Design review of the part built by this model. Coordinates are the model's own, in mm. A direction names the side the tool comes from. Coordinates: 2 decimals unless noted, no trailing zeros. Loops run counter-clockwise (first coordinate to the right, second up) from the corner with the lowest first, then second, coordinate; pieces in that order, holes last.
from build123d import *

# Parameters (mm, degrees)
BOSS_EXTRUDE1_DEPTH      = 7.62
BOSS_EXTRUDE2_DEPTH      = 31.75
BOSS_EXTRUDE2_DEPTH_BACK = 38.1
SKETCH2_W                = 25.4
SKETCH2_H                = 6.985
BOSS_EXTRUDE3_START      = -7.62
BOSS_EXTRUDE3_DEPTH      = 7.62
SKETCH4_R                = 3.175
CUT_EXTRUDE1_DEPTH       = 7.62
CHAMFER1_SIZE            = 8.89
FILLET1_R                = 6.35
FILLET2_R                = 5.08


with BuildPart() as part:
    # Sketch1 → Boss-Extrude1 (new body)
    with BuildSketch(Plane.XY):
        with BuildLine():
            Line((41.275, -41.275), (0, -41.275))
            ThreePointArc((0, -41.275), (-40.972302797, -4.989592018), (-9.906, 40.068650951))
            Line((-9.906, 40.068650951), (-9.906, 0))
            ThreePointArc((-9.906, 0), (0, -9.906), (9.906, 0))
            Line((9.906, 0), (9.906, 40.068650951))
            ThreePointArc((9.906, 40.068650951), (32.4999675, 25.443618797), (41.275, 0))
            Line((41.275, 0), (41.275, -41.275))
        make_face()
    extrude(amount=BOSS_EXTRUDE1_DEPTH)

    # Sketch2 → Boss-Extrude2 (add, two sides: drawn at the far end of the back side and taken through both)
    with BuildSketch(Plane.XY.offset(7.62).offset(-BOSS_EXTRUDE2_DEPTH_BACK)):
        with Locations((28.575, -41.5925)):
            Rectangle(SKETCH2_W, SKETCH2_H)
    extrude(amount=BOSS_EXTRUDE2_DEPTH + BOSS_EXTRUDE2_DEPTH_BACK)

    # Sketch3 → Boss-Extrude3 (add)
    with BuildSketch(Plane.XY.offset(7.62).offset(BOSS_EXTRUDE3_START)):
        with BuildLine():
            Line((15.875, -45.085), (-7.79603534, -40.532054697))
            ThreePointArc((-7.79603534, -40.532054697), (-3.915677934, -41.088843879), (0, -41.275))
            Line((0, -41.275), (15.875, -41.275))
            Line((15.875, -41.275), (15.875, -45.085))
        make_face()
    extrude(amount=BOSS_EXTRUDE3_DEPTH)

    # Sketch4 → Cut-Extrude1 (cut)
    with BuildSketch(Plane(origin=(0, -38.1, 0), x_dir=(1, 0, 0), z_dir=(0, 1, 0))):
        with Locations(Location((28.575, -26.67, 0), (0, 0, 270))):
            Circle(SKETCH4_R)
        with Locations(Location((28.575, 17.78, 0), (0, 0, 270))):
            Circle(SKETCH4_R)
    extrude(amount=-CUT_EXTRUDE1_DEPTH, mode=Mode.SUBTRACT)

    # Chamfer1
    chamfer1_edges = [part.edges().sort_by_distance(p)[0] for p in [
        (28.575, -38.1, 0),
    ]]
    chamfer(chamfer1_edges, length=CHAMFER1_SIZE)

    # Fillet1
    fillet1_edges = [part.edges().sort_by_distance(p)[0] for p in [
        (15.875, -37.1475, 0),
        (15.875, -41.5925, 7.62),
    ]]
    fillet(fillet1_edges, radius=FILLET1_R)

    # Fillet2
    fillet2_edges = [part.edges().sort_by_distance(p)[0] for p in [
        (9.906, 40.068650951, 3.81),
        (-9.906, 40.068650951, 3.81),
    ]]
    fillet(fillet2_edges, radius=FILLET2_R)


solid = part.part
Q1. Take a section at B-B, the plane y = 14. Write out the cut boundary in (x, z), then the cut area to 3 significant figures.
Q2. Take a section at D-D, the plane y = -14. Write out the cut boundary in (x, z) (3 decimals), then the cut area to 3 significant figures.
Q3. Clearance check with flat-ended pins moving along their axes: pin 1 Ø8.5 at (y, z) = (20, 4) entering from +X; pin 2 Ø10 at (x, z) = (28.575, -17.78) entering from +Y; pin 3 Ø6 at (y, z) = (8.5, 4.5) entering from -X. State where each tip first meets the part, or that it passes through.
Q4. Take a section at A-A, the plane z = -17.78. Write out the cut boundary in (x, y) (3 decimals).
Q5. Take a section at C-C, the plane x = 0. Write out the cut boundary in (y, z).
Q6. The part is to be moulded in two halves that separate along X. For faces 1 (the cylindrical face through (-40.893, -5.6, 3.757)), 2 (the cylindrical face through (12.3, 37.26, 3.86)), 3 (the flat face through (1, -11, 7.62)), say which applies: pulls with the +X half, pulls with the -X half, needs draft (parallel to the pull), parting line crosses it, or undercut.
Q7. Machinability: for faces 4 (the flat face through (1, -11, 0)), 5 (the flat face through (28, -38.1, -22)), 6 (the flat face through (15.875, -41, -19)), 7 (the flat face through (-9.906, 17, 4)), which of the approach directions +Z, -Z, +X, -X, +Y, -Y give a long, thin tool a straight path to every point of the face, cutting with its end or side? Answer none if there is none.
Q8. For line 1 (X direction, y = -41.5, z = -17.78) (3 decimals); line 2 (Z direction, x = -19, y = -31); line 3 (Y direction, x = 16, z = -27) (3 decimals), list the stretches that pass through material, from the lowest coordinate up.
Entries:
1. outline: (-38.83, 0) - (-9.91, 0) - (-9.91, 7.62) - (-38.83, 7.62) - close; (9.91, 0) - (38.83, 0) - (38.83, 7.62) - (9.91, 7.62) - close
1. area: 441 mm2
2. outline: (-38.828, 0) - (41.275, 0) - (41.275, 7.62) - (-38.828, 7.62) - close
2. area: 610 mm2
3. pin 1: stops at x = 38.15
3. pin 2: stops at y = -38.1
3. pin 3: stops at x = -40.91
4. outline: (15.875, -45.085) - (25.4, -45.085) - (25.4, -38.1) - (15.875, -38.1) - close; (31.75, -45.085) - (41.275, -45.085) - (41.275, -38.1) - (31.75, -38.1) - close
5. outline: (-42.03, 0) - (-9.91, 0) - (-9.91, 7.62) - (-42.03, 7.62) - close
6. face 1: pulls with the -X half
6. face 2: undercut
6. face 3: needs draft
7. face 4: -Z, -X, +Y
7. face 5: -Z, +X, -X, +Y
7. face 6: -Z, -X, +Y, -Y
7. face 7: +Z, -Z, +Y
8. line 1: x = 15.875 to 25.4, 31.75 to 41.275
8. line 2: z = 0 to 7.62
8. line 3: y = -45.085 to -38.1
